Source: CAD feature listing. Evaluate the final solid. Frame: model axes, mm. Face numbers are marked on the shaded views. A direction names the side the tool comes from. Round coordinates to 2 decimals unless told otherwise and drop trailing zeros. Use a Markdown table: item, result.
Autodesk Fusion 360 part; units mm, degrees
sketch "Sketch1" plane through (0, 0, 0) normal (0, 0, 1) x (1, 0, 0)
  arc A0 (40.8125, 70.866) -> (39.0316, 71.3876) centre (39.6043, 70.0419) ccw
  arc A1 (40.3994, 70.5843) -> (39.3219, 70.962) centre (39.6043, 70.0419) ccw
  arc A2 (45.3863, 40.2197) -> (40.8125, 70.866) centre (11.4188, 50.8147) ccw
  arc A3 (44.9039, 40.3524) -> (40.3994, 70.5843) centre (11.4188, 50.8147) ccw
  line L0 (37.8087, 8.5202) -> (45.3863, 40.2197)
  line L1 (37.3224, 8.6365) -> (44.9039, 40.3524)
  arc A4 (34.9504, 6.3921) -> (37.3224, 8.6365) centre (34.4176, 9.3308) ccw
  arc A5 (35.8752, 6.1635) -> (37.8087, 8.5202) centre (34.4176, 9.3308) ccw
  arc A6 (46.5621, 6.4278) -> (47.4142, 3.3103) centre (49.8315, 5.6462) ccw
  line L2 (54.6994, 40.4687) -> (46.5621, 6.4278)
  arc A7 (55.1857, 40.3524) -> (48.5945, 76.1714) centre (11.4188, 50.8147) ccw
  line L3 (55.1857, 40.3524) -> (47.0484, 6.3115)
  arc A8 (47.0484, 6.3115) -> (49.4188, 2.8147) centre (49.8315, 5.6462) ccw
  arc A9 (54.6994, 40.4687) -> (48.18, 75.8919) centre (11.4188, 50.8147) ccw
  line L4 (39.0316, 71.3876) -> (39.3219, 70.962)
  line L5 (49.4188, 2.8147) -> (47.4142, 3.3103)
  line L6 (34.9504, 6.3921) -> (35.8752, 6.1635)
  line L7 (35.8752, 6.1635) -> (47.4142, 3.3103)
  line L8 (48.18, 75.8919) -> (48.5945, 76.1714)
  line L9 (48.5945, 76.1714) -> (40.7846, 70.9055)
  dimension "d1" = 35
  dimension "d2" = 10
  dimension "d3" = 0.5
  dimension "d4" = 0.5
extrude "Extrude1" add sketch "Sketch1" along normal blind 10.5 contours A0 A1 A2 A3 L0 L1 A4 A5 L4 L6 | A0 A2 L0 A5 A6 L2 A9 L7 L9 | A6 L2 A7 L3 A8 A9 L5 L8 L9
extrude "Extrude2" cut sketch "Sketch1" along normal blind 10 contours A0 A1 A2 A3 L0 L1 A4 A5 L4 L6 | A0 A2 L0 A5 A6 L2 A9 L7 L9 | A6 L2 A7 L3 A8 A9 L5 L8 L9
extrude "Extrude3" add sketch "Sketch1" along normal blind 10 contours A0 A1 A2 A3 L0 L1 A4 A5 L4 L6 | A6 L2 A7 L3 A8 A9 L5 L8 L9
fillet "Fillet1" radius 0.2 8 faces at (49.046, 29.0055, 10.5) (39.8496, 19.2085, 3.5) (36.0166, 6.8083, 7) (46.4714, 52.2383, 7) (40.0271, 70.9065, 7) (52.4733, 29.0055, 7) (54.7333, 63.0152, 7) (48.3714, 3.1853, 7)
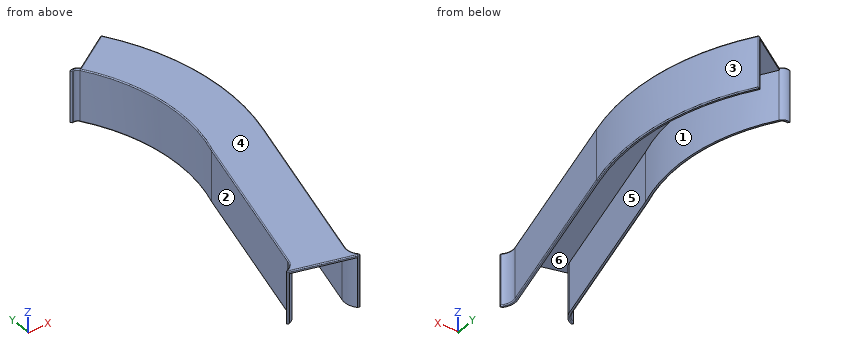
Q1. Reachability of the marked faces 1, 2 and 3 from +Z, -Z, +X, -X, +Y, -Y: full face, straight path, thin tool, end or side. Return the list, or none.
Results are:
| item | result |
|---|---|
| face 1 | -Z |
| face 2 | +Z, -Z, -X |
| face 3 | +Z, -Z, +X |
Q2. Mould query, pull axis Y, two halves, no side actions, for the marked faces 4, 5 and 6. Classes: +Y half, -Y half, draft (parallel to the pull), parting line (faces both ways), or undercut.
Results are:
| item | result |
|---|---|
| face 4 | draft |
| face 5 | -Y half |
| face 6 | undercut |
Q3. Line query: L1, parallel to Z at x = 51.75, y = 56; L2, parallel to X at y = 67, z = 4.5; L3, parallel to X at y = 42.5, z = 1. Output: solid intervals per line, ascending.
Results are:
| item | result |
|---|---|
| L1 | 10 to 10.5 |
| L2 | 42.54 to 43.11, 52.87 to 53.41 |
| L3 | 45.5 to 46.02, 55.14 to 55.64 |
Q4. First-contact query: pin 1 Ø5 at (y, z) = (35, 6) entering from -X; pin 2 Ø4 at (x, y) = (45.5, 21) entering from -Z. Flat tips, straight axial feed; report the tip coordinate or a pass-through.
Results are:
| item | result |
|---|---|
| pin 1 | x = 43.03 |
| pin 2 | z = 10 |
